from build123d import *

# Parameters (mm, degrees)
SKETCH1_R           = 1.5
SKETCH1_R_2         = 1.4999995
BOSS_EXTRUDE1_DEPTH = 1.6


with BuildPart() as part:
    # Sketch1 → Boss-Extrude1 (new body)
    with BuildSketch(Plane.XY.offset(1.6)):
        with BuildLine():
            Line((0, 50.9476), (0, 3))
            ThreePointArc((0, 3), (0.878679656, 0.878679656), (3, 0))
            Line((3, 0), (59.5, 0))
            ThreePointArc((59.5, 0), (60.560660172, 0.439339828), (61, 1.5))
            ThreePointArc((61, 1.5), (70.25, 10.75), (79.5, 1.5))
            ThreePointArc((79.5, 1.5), (79.939339828, 0.439339828), (81, 0))
            Line((81, 0), (83.1, 0))
            ThreePointArc((83.1, 0), (85.221320344, 0.878679656), (86.1, 3))
            Line((86.1, 3), (86.1, 50.9476))
            ThreePointArc((86.1, 50.9476), (85.221320344, 53.068920344), (83.1, 53.9476))
            Line((83.1, 53.9476), (3, 53.9476))
            ThreePointArc((3, 53.9476), (0.878679656, 53.068920344), (0, 50.9476))
        make_face()
        with Locations((3.302, 50.3904)):
            Circle(SKETCH1_R, mode=Mode.SUBTRACT)
        with Locations((3.302, 3.556)):
            Circle(SKETCH1_R, mode=Mode.SUBTRACT)
        with Locations((82.55, 3.556)):
            Circle(SKETCH1_R, mode=Mode.SUBTRACT)
        with Locations((82.55, 50.3904)):
            Circle(SKETCH1_R, mode=Mode.SUBTRACT)
        with Locations((27.4096, 3.556)):
            Circle(SKETCH1_R_2, mode=Mode.SUBTRACT)
        with Locations((56.515, 3.556)):
            Circle(SKETCH1_R, mode=Mode.SUBTRACT)
        with Locations((43.05, 50.3904)):
            Circle(SKETCH1_R, mode=Mode.SUBTRACT)
    extrude(amount=-BOSS_EXTRUDE1_DEPTH)


solid = part.part
Geometry check sheet. Reference: the model listing, model coordinates, mm. Round coordinates to 2 decimals unless told otherwise and drop trailing zeros. Order: outer loops, then holes, each group sorted by start corner. A loop starts at its lowest first (then second) coordinate and runs counter-clockwise, first axis right, second up. Notation, with made-up numbers: (7, 8.25) -> (41, 8.25) arc R9 cw to (41, 23.25) -> close; hole circle Ø1 at (-4.5, 29.5). An arc over 180 degrees is marked (long way). Use one line per item in the form item = value.
1. Cross-section at B-B, the plane z = 0.6. Enter the section's corners in (x, y) (3 decimals), plus the area to 3 significant figures.
Working result:
outline = (0, 3) arc R3 ccw to (3, 0) -> (59.5, 0) arc R1.5 ccw to (61, 1.5) arc R9.25 cw to (79.5, 1.5) arc R1.5 ccw to (81, 0) -> (83.1, 0) arc R3 ccw to (86.1, 3) -> (86.1, 50.948) arc R3 ccw to (83.1, 53.948) -> (3, 53.948) arc R3 ccw to (0, 50.948) -> close; hole circle Ø3 at (3.302, 3.556); hole circle Ø3 at (3.302, 50.39); hole circle Ø3 at (27.41, 3.556); hole circle Ø3 at (43.05, 50.39); hole circle Ø3 at (56.515, 3.556); hole circle Ø3 at (82.55, 3.556); hole circle Ø3 at (82.55, 50.39)
area = 4,420 mm^2
2. Scan lines: line 1 along Y through (x, z) = (82.55, 0.4); line 2 along Y through (x, z) = (43.05, 1.15); line 3 along X through (y, z) = (50, 1.3). Record each from-to range of solid material in increasing order. Write a range as from..to.
Working result:
line_1 = 0..2.06, 5.06..48.89, 51.89..53.95
line_2 = 0..48.89, 51.89..53.95
line_3 = 0..1.85, 4.75..41.6, 44.5..81.1, 84..86.1
3. Mould release check, pull along Y, two halves, no side actions. Record for faces 1 (the face through (4.733, 50.841, 0.811)), 2 (the face through (0, 27, 1)), 3 (the face through (31, 0, 1)): pulls with the +Y half, pulls with the -Y half, needs draft (parallel to the pull), parting line crosses it, or undercut.
Working result:
face_1 = undercut
face_2 = needs draft
face_3 = pulls with the -Y half
4. Cross-section at C-C, the plane x = 70.25. Enter the section's corners in (y, z).
Working result:
outline = (10.75, 0) -> (53.95, 0) -> (53.95, 1.6) -> (10.75, 1.6) -> close
5. Go/stop test with a flat-tipped pin: pin 1 (1.8 mm diameter, centred on x = 82.55, y = 3.556, fed in from +Z). Record where the tip stops, or that it passes through.
Working result:
pin_1 = through
6. Cross-section at A-A, the plane x = 43.05. Enter the section's corners in (y, z).
Working result:
outline = (0, 0) -> (48.89, 0) -> (48.89, 1.6) -> (0, 1.6) -> close; (51.89, 0) -> (53.95, 0) -> (53.95, 1.6) -> (51.89, 1.6) -> close
